Input: part model. Units: mm. Frame: model coordinates. Coordinates: 2 decimals unless noted, no trailing zeros. Loops run counter-clockwise (first coordinate to the right, second up) from the corner with the lowest first, then second, coordinate; pieces in that order, holes last.
(1) Line query: L1, parallel to X at y = -4.5, z = 0.95; L2, parallel to X at y = 0.5, z = 0.5; L3, parallel to Y at x = 32, z = 0.25. Output: solid intervals per line, ascending.
(2) Section B-B, the plane x = -26. Return loops of the section in (y, z), then the cut area to 3 significant figures.
(3) Section C-C, the plane y = -4.5. Return loops of the section in (x, z), then the cut area to 3 significant figures.
(4) Section A-A, the plane z = 1.1. Return loops of the section in (x, y), then the cut area to 3 significant figures.
```python
from build123d import *

# Parameters (mm, degrees)
SKETCH1_W               = 77
SKETCH1_H               = 11
BOSS_EXTRUDE1_DEPTH     = 1.6
CUT_EXTRUDE1_DEPTH      = 39.923771657
CUT_EXTRUDE1_DEPTH_BACK = 10
FILLET2_R               = 1


with BuildPart() as part:
    # Sketch1 → Boss-Extrude1 (new body)
    with BuildSketch(Plane.XY):
        Rectangle(SKETCH1_W, SKETCH1_H)
    extrude(amount=BOSS_EXTRUDE1_DEPTH)

    # Sketch2 → Cut-Extrude1 (cut, two sides: drawn at the far end of the back side and taken through both)
    with BuildSketch(Plane.XY.offset(1.6).offset(-CUT_EXTRUDE1_DEPTH_BACK)):
        Polygon((38.5, -5.5), (38.5, 5.5), (24.04554885, -5.5), align=None)
        Polygon((-38.5, -5.5), (-24.04554885, 5.5), (-38.5, 5.5), align=None)
    extrude(amount=CUT_EXTRUDE1_DEPTH + CUT_EXTRUDE1_DEPTH_BACK, mode=Mode.SUBTRACT)

    # Fillet2
    fillet2_edges = [part.edges().sort_by_distance(p)[0] for p in [
        (24.04554885, -5.5, 0.8),
        (-24.04554885, 5.5, 0.8),
        (-38.5, -5.5, 0.8),
        (38.5, 5.5, 0.8),
    ]]
    fillet(fillet2_edges, radius=FILLET2_R)


solid = part.part
```
Report:
1. L1: x = -36.53 to 25.36
1. L2: x = -30.62 to 31.93
1. L3: y = 0.55 to 5.5
2. outline: (-5.5, 0) - (4.01, 0) - (4.01, 1.6) - (-5.5, 1.6) - close
2. area: 15.2 mm2
3. outline: (-36.53, 0) - (25.36, 0) - (25.36, 1.6) - (-36.53, 1.6) - close
3. area: 99.0 mm2
4. outline: (-36.14, -3.7) arc R1 ccw to (-35.53, -5.5) - (23.71, -5.5) arc R1 ccw to (24.31, -5.3) - (36.14, 3.7) arc R1 ccw to (35.53, 5.5) - (-23.71, 5.5) arc R1 ccw to (-24.31, 5.3) - close
4. area: 685 mm2
